Read the model definition and answer for the solid it produces. Units are mm, in the model's axes. Face numbers are marked on the shaded views. A direction names the side the tool comes from. Coordinates: 2 decimals unless noted, no trailing zeros. Order: outer loops, then holes, each group sorted by start corner. A loop starts at its lowest first (then second) coordinate and runs counter-clockwise, first axis right, second up. Notation, with made-up numbers: M 35.25,42.25 L 47.25,42.25 A27 ccw 47.25,61.25 Z; hole C 23.25,22 d2. An arc over 180 degrees is marked long. Put each result on its own line as item: value.
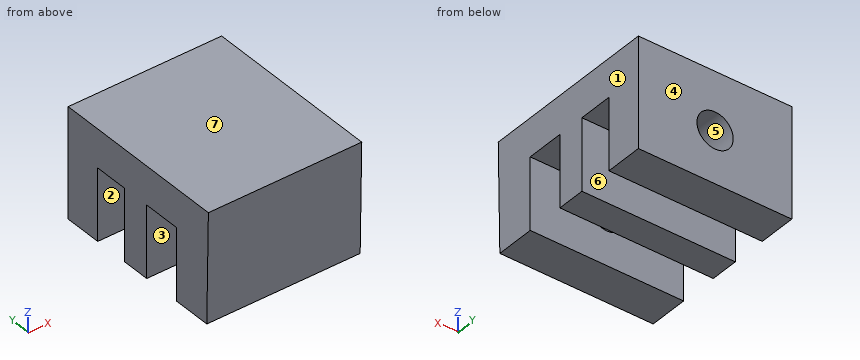
from build123d import *

# Parameters (mm, degrees)
BOSS_EXTRUDE1_DEPTH = 50
SKETCH2_R           = 11.83848923
CUT_EXTRUDE1_DEPTH  = 100.430977097


with BuildPart() as part:
    # Sketch1 → Boss-Extrude1 (new, symmetric)
    with BuildSketch(Plane(origin=(0, 0, 0), x_dir=(0, 0, -1), z_dir=(1, 0, 0))):
        Polygon((0, 53.746712803), (0, -49.386309295), (71.662283737, -48.059229966), (71.662283737, -22.655139964), (24.835341718, -22.655139964), (24.835341718, 2.180201754), (71.662283737, 2.180201754), (71.662283737, 20.569729591), (24.835341718, 20.569729591), (24.835341718, 43.130078175), (71.662283737, 43.130078175), (71.662283737, 67.775837132), (0, 67.775837132), align=None)
    extrude(amount=BOSS_EXTRUDE1_DEPTH, both=True)

    # Sketch2 → Cut-Extrude1 (cut)
    with BuildSketch(Plane(origin=(0, 67.775837132, 0), x_dir=(1, 0, 0), z_dir=(0, 1, 0))):
        with Locations(Location((0, 37.695226778, 0), (0, 0, 270))):
            Circle(SKETCH2_R)
    extrude(amount=-CUT_EXTRUDE1_DEPTH, mode=Mode.SUBTRACT)


solid = part.part
Q1. Consider line 1 along Y through (x, z) = (-23, -39.5); line 2 along Y through (x, z) = (-6, -52.5); line 3 along X through (y, z) = (51, -28). Determine where each line is inside the solid, lowest interval first.
Answers below:
line 1: y = -48.65 to -22.66, 2.18 to 20.57, 43.13 to 67.78
line 2: y = -48.41 to -22.66, 2.18 to 20.57, 43.13 to 67.78
line 3: x = -50 to -6.79, 6.79 to 50
Q2. Given pin 1 (5 mm diameter, centred on x = -26, y = -11, fed in from -Z); pin 2 (3 mm diameter, centred on x = 24.5, z = -18, fed in from -Y); pin 3 (19 mm diameter, centred on x = -4, z = -38.5, fed in from +Y); pin 4 (23.5 mm diameter, centred on x = -1.5, z = -54.5, fed in from -Y), each flat-ended and moving along its own axis, determine where each tip first touches the part or whether it passes through.
Answers below:
pin 1: stops at z = -24.84
pin 2: stops at y = -49.08
pin 3: stops at y = 67.78
pin 4: stops at y = -48.59
Q3. For a pull along Y with two mould halves and no side action, classify the marked faces 1, 2, 3 and 4 as +Y half, -Y half, draft (parallel to the pull), parting line (faces both ways), or undercut.
Answers below:
face 1: draft
face 2: undercut
face 3: undercut
face 4: +Y half
Q4. Find section A-A on x = 0. Write down the section's boundary in (y, z).
Answers below:
outline: M -49.39,0 L -48.06,-71.66 L -22.66,-71.66 L -22.66,-49.53 L -32.66,-49.53 L -32.66,-25.86 L -22.66,-25.86 L -22.66,-24.84 L 2.18,-24.84 L 2.18,-25.86 L 20.57,-25.86 L 20.57,-24.84 L 43.13,-24.84 L 43.13,-25.86 L 67.78,-25.86 L 67.78,0 Z; M 2.18,-71.66 L 20.57,-71.66 L 20.57,-49.53 L 2.18,-49.53 Z; M 43.13,-71.66 L 67.78,-71.66 L 67.78,-49.53 L 43.13,-49.53 Z
Q5. Find section D-D on z = -29.5. Write down the section's boundary in (x, y).
Answers below:
outline: M -50,-48.84 L 50,-48.84 L 50,-22.66 L 8.54,-22.66 L 8.54,-32.66 L -8.54,-32.66 L -8.54,-22.66 L -50,-22.66 Z; M -50,2.18 L -8.54,2.18 L -8.54,20.57 L -50,20.57 Z; M -50,43.13 L -8.54,43.13 L -8.54,67.78 L -50,67.78 Z; M 8.54,2.18 L 50,2.18 L 50,20.57 L 8.54,20.57 Z; M 8.54,43.13 L 50,43.13 L 50,67.78 L 8.54,67.78 Z
Q6. Find section B-B on z = -59.5. Write down the section's boundary in (x, y).
Answers below:
outline: M -50,-48.28 L 50,-48.28 L 50,-22.66 L -50,-22.66 Z; M -50,2.18 L 50,2.18 L 50,20.57 L -50,20.57 Z; M -50,43.13 L 50,43.13 L 50,67.78 L -50,67.78 Z
Q7. Find section C-C on y = -30. Write down the section's boundary in (x, z), plus the area to 3 significant figures.
Answers below:
outline: M -50,-71.66 L 50,-71.66 L 50,0 L -50,0 Z; hole C 0,-37.7 d23.68
area: 6,730 mm^2
Q8. A tool of negligible diameter and unlimited length cuts with its end or side. For the marked faces 5, 6 and 7, from which of +Z, -Z, +X, -X, +Y, -Y can it reach the whole face along a straight path? Write none if from no direction.
Answers below:
face 5: +Y
face 6: -Z, +X, -X
face 7: +Z, +X, -X, +Y, -Y
